from build123d import *

# Parameters (mm, degrees)
BOSS_EXTRUDE1_DEPTH = 3.175
FILLET1_R           = 3.81
CUT_EXTRUDE1_DEPTH  = 3.175
FILLET2_R           = 6.35
SKETCH5_W           = 259.08
SKETCH5_H           = 3.175
BOSS_EXTRUDE2_DEPTH = 4.7625
CUT_EXTRUDE2_REACH  = 360.417
SKETCH6_W           = 50.8
SKETCH6_H           = 4.7879
SKETCH9_W           = 259.08
SKETCH9_H           = 3.175
BOSS_EXTRUDE3_DEPTH = 4.7625
SKETCH10_R          = 3.175
CUT_EXTRUDE4_DEPTH  = 359.417423579


with BuildPart() as part:
    # Sketch2 → Boss-Extrude1 (new body)
    with BuildSketch(Plane(origin=(0, 0, 0), x_dir=(1, 0, 0), z_dir=(0, 1, 0))):
        Polygon((0, 0), (259.08, 0), (160.02, -247.65), (99.06, -247.65), align=None)
        Polygon((152.079282437, -235.710784307), (106.359282437, -235.710784307), (129.772405457, -143.63904611), align=None, mode=Mode.SUBTRACT)
        Polygon((101.296371264, -209.241791453), (122.57344543, -125.570031796), (67.827667402, -125.570031796), align=None, mode=Mode.SUBTRACT)
        Polygon((157.226545347, -208.413887274), (190.364087539, -125.570031796), (137.155373359, -125.570031796), align=None, mode=Mode.SUBTRACT)
    extrude(amount=BOSS_EXTRUDE1_DEPTH)

    # Fillet1
    fillet1_edges = [part.edges().sort_by_distance(p)[0] for p in [
        (152.079282437, 1.5875, 235.710784307),
        (129.772405457, 1.5875, 143.63904611),
        (106.359282437, 1.5875, 235.710784307),
        (67.827667402, 1.5875, 125.570031796),
        (101.296371264, 1.5875, 209.241791453),
        (122.57344543, 1.5875, 125.570031796),
        (137.155373359, 1.5875, 125.570031796),
        (157.226545347, 1.5875, 208.413887274),
        (190.364087539, 1.5875, 125.570031796),
    ]]
    fillet(fillet1_edges, radius=FILLET1_R)

    # Sketch3 → Cut-Extrude1 (cut)
    with BuildSketch(Plane(origin=(0, 3.175, 0), x_dir=(1, 0, 0), z_dir=(0, 1, 0))):
        Polygon((167.64, -25.4), (228.402522085, -25.4), (195.954509366, -106.520031796), (167.64, -106.520031796), align=None)
        Polygon((91.44, -106.520031796), (91.44, -25.4), (30.677477915, -25.4), (63.125490634, -106.520031796), align=None)
    extrude(amount=-CUT_EXTRUDE1_DEPTH, mode=Mode.SUBTRACT)

    # Fillet2
    fillet2_edges = [part.edges().sort_by_distance(p)[0] for p in [
        (195.954509366, 1.5875, 106.520031796),
        (228.402522085, 1.5875, 25.4),
        (167.64, 1.5875, 25.4),
        (167.64, 1.5875, 106.520031796),
        (91.44, 1.5875, 25.4),
        (30.677477915, 1.5875, 25.4),
        (63.125490634, 1.5875, 106.520031796),
        (91.44, 1.5875, 106.520031796),
    ]]
    fillet(fillet2_edges, radius=FILLET2_R)

    # Sketch5 → Boss-Extrude2 (add)
    with BuildSketch(Plane(origin=(0, 0, 0), x_dir=(-1, 0, 0), z_dir=(0, 0, -1))):
        with Locations((-129.54, 1.5875)):
            Rectangle(SKETCH5_W, SKETCH5_H)
    extrude(amount=BOSS_EXTRUDE2_DEPTH)

    # Sketch6 → Cut-Extrude2 (cut, up to next)
    with BuildSketch(Plane(origin=(0, 3.175, 0), x_dir=(1, 0, 0), z_dir=(0, 1, 0)), mode=Mode.PRIVATE) as cut_extrude2_sk1:
        with Locations((129.526089834, -119.84355)):
            Rectangle(SKETCH6_W, SKETCH6_H)
    cut_extrude2_tool1 = extrude(cut_extrude2_sk1.sketch, amount=-CUT_EXTRUDE2_REACH, mode=Mode.PRIVATE) & part.part
    add(cut_extrude2_tool1.solids().sort_by_distance((129.52609, 3.175, 119.84355))[0], mode=Mode.SUBTRACT)

    # Sketch9 → Boss-Extrude3 (add)
    with BuildSketch(Plane(origin=(0, 0, -4.7625), x_dir=(-1, 0, 0), z_dir=(0, 0, -1))):
        with Locations((-129.54, 1.5875)):
            Rectangle(SKETCH9_W, SKETCH9_H)
    extrude(amount=BOSS_EXTRUDE3_DEPTH)

    # Sketch10 → Cut-Extrude4 (cut, through all)
    with BuildSketch(Plane(origin=(0, 3.175, 0), x_dir=(1, 0, 0), z_dir=(0, 1, 0))):
        with Locations(Location((99.822, -98.3996, 0), (0, 0, 270))):
            Circle(SKETCH10_R)
        with Locations(Location((159.258, -98.3996, 0), (0, 0, 270))):
            Circle(SKETCH10_R)
        with Locations(Location((99.822, -9.525, 0), (0, 0, 270))):
            Circle(SKETCH10_R)
        with Locations(Location((159.258, -9.525, 0), (0, 0, 270))):
            Circle(SKETCH10_R)
    extrude(amount=-CUT_EXTRUDE4_DEPTH, mode=Mode.SUBTRACT)


solid = part.part
Build history of the part. All positions in model axes, mm. A direction names the side the tool comes from. Round coordinates to 2 decimals unless told otherwise and drop trailing zeros. Loops run counter-clockwise (first coordinate to the right, second up) from the corner with the lowest first, then second, coordinate; pieces in that order, holes last. Notation, with made-up numbers: (-0.5, 60.5) -> (10.5, 60.5) arc R22 ccw to (10.5, 96.5) -> close; hole circle Ø5 at (-8.5, -30). An arc over 180 degrees is marked (long way). Answer in a Markdown table with one row per item.
Item 1: Mould opens along Z. For faces 1 (the flat face through (210.243, 1.565, 122.091)), 2 (the flat face through (116.65, 1.57, 195.24)), 3 (the flat face through (131, 0, 92)) say: +Z half, -Z half, draft (parallel to the pull), parting line (faces both ways), or undercut.
Answers below:
| item | result |
|---|---|
| face 1 | +Z half |
| face 2 | undercut |
| face 3 | draft |
Item 2: Saw through at A-A (x = 52). Write the cut outline in (y, z) (3 decimals), and give its area (3 significant figures).
Answers below:
| item | result |
|---|---|
| outline | (0, -9.525) -> (3.175, -9.525) -> (3.175, 25.4) -> (0, 25.4) -> close; (0, 78.706) -> (3.175, 78.706) -> (3.175, 130) -> (0, 130) -> close |
| area | 274 mm² |
Item 3: Saw through at D-D (y = 0.5). State how many separate pieces and enclosed holes the cut face has, and give its area (3 significant figures).
Answers below:
| item | result |
|---|---|
| separate pieces | 1 |
| enclosed holes | 10 |
| area | 28,100 mm² |
Item 4: Drill centre lines: L1, parallel to X at y = 1.9, z = 102; L2, parallel to X at y = 0.95, z = 165.5; L3, parallel to X at y = 2.4, z = 38. Where is each one in solid material? Low to high. Write a range as [from, to].
Answers below:
| item | result |
|---|---|
| L1 | x = [40.8, 61.32], [91.17, 167.91], [197.76, 218.28] |
| L2 | x = [66.2, 83.8], [112.42, 124.21], [135.07, 146.83], [174.39, 192.88] |
| L3 | x = [15.2, 35.72], [91.44, 167.64], [223.36, 243.88] |
Item 5: Saw through at C-C (z = 62). Write the cut outline in (x, y) (3 decimals).
Answers below:
| item | result |
|---|---|
| outline | (24.8, 0) -> (45.317, 0) -> (45.317, 3.175) -> (24.8, 3.175) -> close; (91.44, 0) -> (167.64, 0) -> (167.64, 3.175) -> (91.44, 3.175) -> close; (213.763, 0) -> (234.28, 0) -> (234.28, 3.175) -> (213.763, 3.175) -> close |
Item 6: Saw through at B-B (z = 193.5). Write the cut outline in (x, y) (3 decimals).
Answers below:
| item | result |
|---|---|
| outline | (77.4, 0) -> (95, 0) -> (95, 3.175) -> (77.4, 3.175) -> close; (105.299, 0) -> (117.093, 0) -> (117.093, 3.175) -> (105.299, 3.175) -> close; (141.853, 0) -> (153.613, 0) -> (153.613, 3.175) -> (141.853, 3.175) -> close; (163.192, 0) -> (181.68, 0) -> (181.68, 3.175) -> (163.192, 3.175) -> close |
Item 7: Pin check, flat tips, straight feed: pin 1 (5 mm diameter, centred on x = 159.258, z = 9.525, fed in from +Y); pin 2 (1.5 mm diameter, centred on y = 0.5, z = 167, fed in from -X); pin 3 (1 mm diameter, centred on y = 1.5, z = 119, fed in from +X); pin 4 (4 mm diameter, centred on x = 134.5, z = 105.5, fed in from -Y). Stop position of each tip, or through.
Answers below:
| item | result |
|---|---|
| pin 1 | passes through |
| pin 2 | stops at x = 66.5 |
| pin 3 | stops at x = 211.68 |
| pin 4 | stops at y = 0 |
Item 8: Which spindle directions (+Z, -Z, +X, -X, +Y, -Y) get a long thin tool onto all of the face, cutting with end or side? Do faces 4 (the flat face through (142.04, 1.57, 194.27)), 5 (the flat face through (131, 3.175, 92)). Say none if no direction does.
Answers below:
| item | result |
|---|---|
| face 4 | +Y, -Y |
| face 5 | +Z, -Z, +X, -X, +Y |
